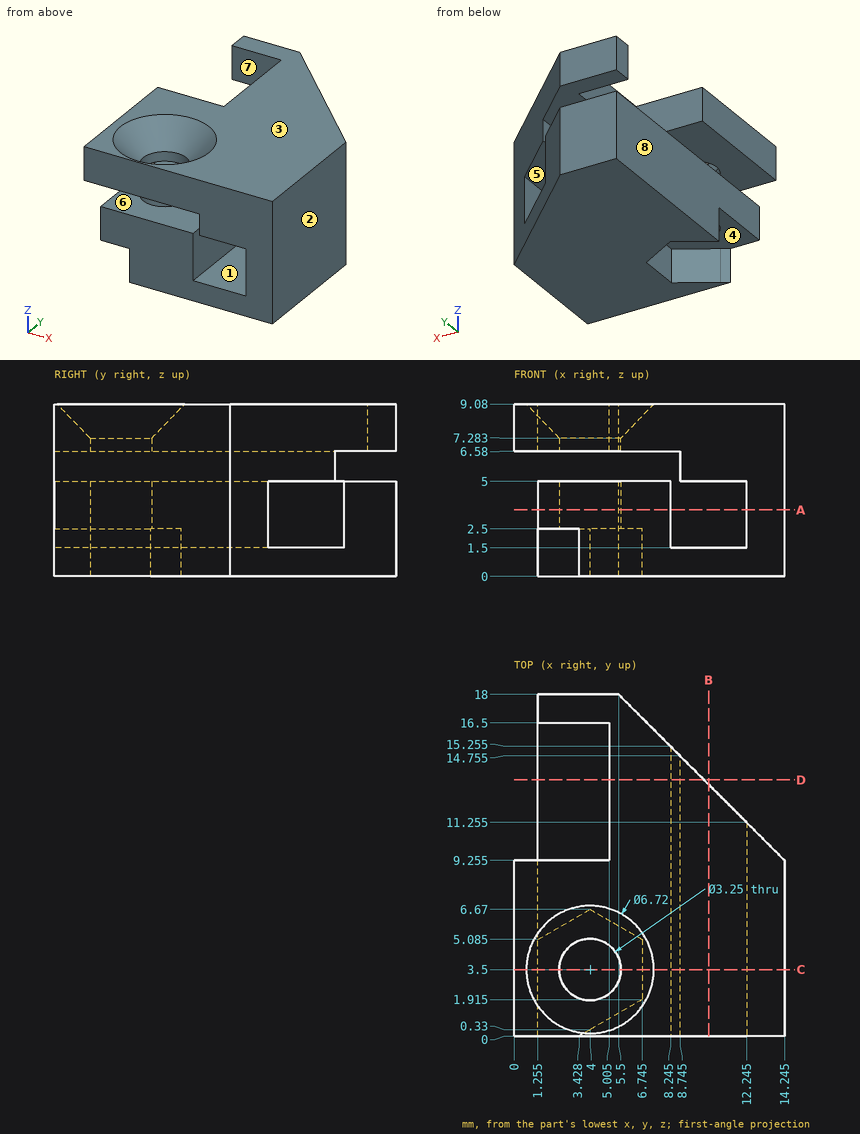
Source: three-view drawing plus pictorial views. Frame: mm from the lowest corner of the part. A direction names the side the tool comes from. Coordinates: 2 decimals unless noted, no trailing zeros. Loops run counter-clockwise (first coordinate to the right, second up) from the corner with the lowest first, then second, coordinate; pieces in that order, holes last. Notation, with made-up numbers: (0.25, 23.25) -> (52.25, 23.25) arc R11 ccw to (52.25, 34.25) -> close; hole circle Ø1 at (-40, 11.25). An arc over 180 degrees is marked (long way). Write each question's results on one line, items separated by ' | '. Start each with the question number.
Q1. Pull-direction query (Z, two-part tool) for the marked faces 1, 2 and 3; classes: released by +Z, released by -Z, zero draft, split by the parting line, or undercut.
Q2. Pin query (flat end, axial travel): pin 1 (4 mm diameter, centred on y = 6.5, z = 3.5, fed in from -X) (1 decimal); pin 2 (5 mm diameter, centred on x = 9, z = 1, fed in from +Y); pin 3 (3 mm diameter, centred on x = 4, y = 3.5, fed in from +Z); pin 4 (2 mm diameter, centred on y = 2.5, z = 1, fed in from -X) (1 decimal). Return the tip coordinate at first contact, or that it passes through.
Q3. Section A-A, the plane z = 3.5. State how many separate pieces and enclosed holes the cut face has, plus the area to 3 significant figures.
Q4. Section B-B, the plane x = 10.25. Return the cut outline in (y, z).
Q5. Ray query, line 1 (Y direction, x = 4, z = 3.5) (1 decimal); line 2 (Z direction, x = 7, y = 5.5); line 3 (Y direction, x = 4, z = 6.85) (1 decimal). Return the intervals inside material, ascending. Write a range as from..to.
Q6. Section D-D, the plane y = 13.5. Return the cut outline in (x, z) (1 decimal).
Q7. Section C-C, the plane y = 3.5. Return the cut outline in (x, z) (1 decimal).
Q8. Reachability of the marked faces 4, 5, 6, 7 and 8 from +Z, -Z, +X, -X, +Y, -Y: full face, straight path, thin tool, end or side. Return the list, or none.
Found:
1) face 1: undercut | face 2: zero draft | face 3: released by +Z
2) pin 1: x = 1.3 | pin 2: y = 17 | pin 3: through | pin 4: x = 6
3) separate pieces: 2 | enclosed holes: 1 | area: 134 mm2
4) outline: (0, 0) -> (13.25, 0) -> (13.25, 1.5) -> (0, 1.5) -> close; (0, 5) -> (13.25, 5) -> (13.25, 9.08) -> (0, 9.08) -> close
5) line 1: 0..1.9, 5.1..18 | line 2: 0..5, 6.58..9.08 | line 3: 0..1.9, 5.1..9.3, 16.5..18
6) outline: (1.3, 0) -> (10, 0) -> (10, 1.5) -> (8.2, 1.5) -> (8.2, 5) -> (1.3, 5) -> close; (5, 6.6) -> (8.7, 6.6) -> (8.7, 5) -> (10, 5) -> (10, 9.1) -> (5, 9.1) -> close
7) outline: (0, 6.6) -> (2.4, 6.6) -> (2.4, 7.3) -> (0.6, 9.1) -> (0, 9.1) -> close; (1.3, 2.5) -> (2.4, 2.5) -> (2.4, 5) -> (1.3, 5) -> close; (5.6, 2.5) -> (6.7, 2.5) -> (6.7, 0) -> (14.2, 0) -> (14.2, 9.1) -> (7.4, 9.1) -> (5.6, 7.3) -> (5.6, 6.6) -> (8.7, 6.6) -> (8.7, 5) -> (12.2, 5) -> (12.2, 1.5) -> (8.2, 1.5) -> (8.2, 5) -> (5.6, 5) -> close
8) face 4: -Z | face 5: +Y, -Y | face 6: -X, +Y, -Y | face 7: +Z, -X | face 8: -Z, -X, +Y, -Y
